The model under review builds one solid part; all positions refer to its coordinate system, in mm. A direction names the side the tool comes from. Round coordinates to 2 decimals unless told otherwise and drop trailing zeros. Write each loop counter-clockwise with the first axis right and the second up, starting at its lowest first coordinate (ties: lowest second). Pieces come first, ordered by that corner, then holes. Notation, with made-up numbers: M 38.25,65 L 63.25,65 A20 cw 63.25,81 Z; hole C 38.25,79.25 d9. An arc over 180 degrees is marked long. Write item = value, one per line. Start each with the question number.
Item 1: Tool access review of faces 1 (the flat face through (0, 0, 0)), 2 (the cylindrical face through (11.61, 20.76, 2.97)): name each direction out of +Z, -Z, +X, -X, +Y, -Y from which nothing blocks a thin tool from reaching the whole face with its end or side.
Item 2: Take a section at D-D, the plane x = -10. Give the boundary of the cut face in (y, z), plus the area to 3 significant figures.
Item 3: To check wall thickness, follow line 1 along X through (y, z) = (-1.5, 2); line 2 along Z through (x, y) = (0, 1.5); line 3 along Y through (x, z) = (-20, 3.75). State the ranges of each line that lie inside material, in increasing order.
Item 4: The part is to be moulded in two halves that separate along X. For faces 3 (the cylindrical face through (-0.26, -0.049, 7.483)), 4 (the flat face through (0, 0, 11)), 5 (the flat face through (25, 0, 5)), say which applies: +X half, -X half, draft (parallel to the pull), parting line (faces both ways), or undercut.
Item 5: Take a section at B-B, the plane y = 0. Give the boundary of the cut face in (x, z), plus the area to 3 significant figures.
Item 6: For pin 1 Ø1 at (y, z) = (31.5, 2.5) entering from -X, flat-tipped, find the tip position at first contact; note if it passes through.
Item 7: Take a section at A-A, the plane z = 5.5. Give the boundary of the cut face in (x, y), plus the area to 3 significant figures.
Item 8: Take a section at C-C, the plane x = 0. Give the boundary of the cut face in (y, z), plus the area to 3 significant figures.
from build123d import *

# Parameters (mm, degrees)
SKETCH1_W           = 50
SKETCH1_H           = 7
BOSS_EXTRUDE1_DEPTH = 11
SKETCH2_R           = 2
CUT_EXTRUDE1_DEPTH  = 12
SKETCH3_R           = 2
CUT_EXTRUDE2_DEPTH  = 8
SKETCH4_R           = 3
BOSS_EXTRUDE2_DEPTH = 35


with BuildPart() as part:
    # Sketch1 → Boss-Extrude1 (new body)
    with BuildSketch(Plane.XY):
        Rectangle(SKETCH1_W, SKETCH1_H)
    extrude(amount=BOSS_EXTRUDE1_DEPTH)

    # Sketch2 → Cut-Extrude1 (cut, through all)
    with BuildSketch(Plane(origin=(0, 0, 0), x_dir=(-1, 0, 0), z_dir=(0, 0, -1))):
        with Locations((20, 0)):
            Circle(SKETCH2_R)
        with Locations((-20, 0)):
            Circle(SKETCH2_R)
    extrude(amount=-CUT_EXTRUDE1_DEPTH, mode=Mode.SUBTRACT)

    # Sketch3 → Cut-Extrude2 (cut, through all)
    with BuildSketch(Plane.XZ.offset(3.5)):
        with Locations((0, 5.5)):
            Circle(SKETCH3_R)
    extrude(amount=-CUT_EXTRUDE2_DEPTH, mode=Mode.SUBTRACT)

    # Sketch4 → Boss-Extrude2 (add)
    with BuildSketch(Plane(origin=(0, 3.5, 0), x_dir=(1, 0, 0), z_dir=(0, 1, 0))):
        with Locations((-10, -5.5)):
            Circle(SKETCH4_R)
        with Locations((10, -5.5)):
            Circle(SKETCH4_R)
    extrude(amount=BOSS_EXTRUDE2_DEPTH)


solid = part.part
Response values:
q1.face_1 = -Z, +X, -X, +Y, -Y
q1.face_2 = +Y
q2.outline = M -3.5,0 L 3.5,0 L 3.5,2.5 L 38.5,2.5 L 38.5,8.5 L 3.5,8.5 L 3.5,11 L -3.5,11 Z
q2.area = 287 mm2
q3.line_1 = -25 to -21.32, -18.68 to 18.68, 21.32 to 25
q3.line_2 = 0 to 3.5, 7.5 to 11
q3.line_3 = -3.5 to -2, 2 to 3.5
q4.face_3 = undercut
q4.face_4 = draft
q4.face_5 = +X half
q5.outline = M -25,0 L -22,0 L -22,11 L -25,11 Z; M -18,0 L 18,0 L 18,11 L -18,11 Z; M 22,0 L 25,0 L 25,11 L 22,11 Z; hole C 0,5.5 d4
q5.area = 449 mm2
q6.pin_1 = -11.66
q7.outline = M -25,-3.5 L -2,-3.5 L -2,3.5 L -7,3.5 L -7,38.5 L -13,38.5 L -13,3.5 L -25,3.5 Z; M 2,-3.5 L 25,-3.5 L 25,3.5 L 13,3.5 L 13,38.5 L 7,38.5 L 7,3.5 L 2,3.5 Z; hole C -20,0 d4; hole C 20,0 d4
q7.area = 717 mm2
q8.outline = M -3.5,0 L 3.5,0 L 3.5,3.5 L -3.5,3.5 Z; M -3.5,7.5 L 3.5,7.5 L 3.5,11 L -3.5,11 Z
q8.area = 49.0 mm2
